```python
from build123d import *

# Parameters (mm, degrees)
F3_D     = 2
F3_DEPTH = 5
F3_TIP   = 0.600860619
F4_W     = 2
F4_H     = 4
F7_D     = 2.5
F7_DEPTH = 6.5
F7_TIP   = 0.7510757738


with BuildPart() as f1:
    # F0 (on Right) → F1 (revolve)
    with BuildSketch(Plane.YZ):
        Polygon((5, 47), (0, 47), (0, 23), (3, 23), (3, 25), (8, 25), (8, 32), (20, 32), (20, 47), (15, 47), (15, 42), (10, 42), align=None)
    revolve(axis=Axis((0, 13.034472242, 0), (0, 1, 0)))

    # F3
    with Locations(Plane(origin=(0, 8, 0), x_dir=(-1, 0, 0), z_dir=(0, 1, 0))):
        with Locations((0, 28.5), (24.6817240079, -14.25), (-24.6817240079, -14.25)):
            Hole(F3_D / 2, depth=F3_DEPTH)
            with Locations((0, 0, -(F3_DEPTH + F3_TIP / 2))):  # 118° drill point
                Cone(0, F3_D / 2, F3_TIP, mode=Mode.SUBTRACT)

    # F4 (on Right) → F5 (revolve)
    with BuildSketch(Plane.YZ):
        with Locations((-1, 45)):
            Rectangle(F4_W, F4_H)
    revolve(axis=Axis((0, -7.9047670588, 0), (0, -1, 0)))

    # F7
    with Locations(Plane.XZ):
        with Locations((0, 37.5), (32.4759526419, -18.75), (-32.4759526419, -18.75)):
            Hole(F7_D / 2, depth=F7_DEPTH)
            with Locations((0, 0, -(F7_DEPTH + F7_TIP / 2))):  # 118° drill point
                Cone(0, F7_D / 2, F7_TIP, mode=Mode.SUBTRACT)


solid = f1.part
```
Source: CAD feature listing. Evaluate the final solid. Frame: model axes, mm. A direction names the side the tool comes from. Coordinates: 2 decimals unless noted, no trailing zeros. Loops run counter-clockwise (first coordinate to the right, second up) from the corner with the lowest first, then second, coordinate; pieces in that order, holes last. Notation, with made-up numbers: (-23.75, -9.5) -> (32.25, -9.5) arc R25 cw to (32.25, 26.5) -> close; hole circle Ø8 at (-34.75, 23.5). An arc over 180 degrees is marked (long way). One line per item, written item: value. Start each with the question number.
Q1. Set-up query: faces 4 (the face through (-14.12, 1.55, 44.83)), 5 (the face through (-31, 20, -10)), 6 (the face through (-33.668, 3.296, -18.375)), 7 (the face through (-31.24, 14.08, -6.94)), 8 (the face through (12.62, 12.46, 40.06)). Return all of +Z, -Z, +X, -X, +Y, -Y with unobstructed straight access to the full face (end or side cutting, diameter ignored); none if empty.
Q2. Section query A-A, the plane z = 0. Return the cut outline in (x, y).
Q3. Mould query, pull axis X, two halves, no side actions, for faces 1 (the face through (-24, 15, -35)), 2 (the face through (12.71, 9.687, 40.359)), 3 (the face through (22.804, 1.521, -2.994)). Classes: pulls with the +X half, pulls with the -X half, needs draft (parallel to the pull), parting line crosses it, or undercut.
Q4. Contact query for flat-ended pins moving along their axis: P1, Ø3, axis at x = 0, z = 37.5, coming from the -Y side; P2, Ø12, axis at x = -36, y = 17.5, coming from the -Z side; P3, Ø1.6, axis at x = 0, z = 28.5, coming from the +Y side; P4, Ø5, axis at x = -15.5, z = -9.5, coming from the +Y side. Output: stop coordinate, or through.
Q5. Line query: line 1 along X through (y, z) = (1.15, 0); line 2 along X through (y, z) = (-0.6, 0); line 3 along X through (y, z) = (5, -18.75). Output: solid intervals per line, ascending.
Results:
1. face 4: +Y, -Y
1. face 5: +Z, -Z, +X, -X, +Y
1. face 6: -Y
1. face 7: +Y
1. face 8: none
2. outline: (-47, -2) -> (-43, -2) -> (-43, 0) -> (-23, 0) -> (-23, 3) -> (-25, 3) -> (-25, 8) -> (-32, 8) -> (-32, 20) -> (-47, 20) -> (-47, 15) -> (-42, 15) -> (-42, 10) -> (-47, 5) -> close; (23, 0) -> (43, 0) -> (43, -2) -> (47, -2) -> (47, 5) -> (42, 10) -> (42, 15) -> (47, 15) -> (47, 20) -> (32, 20) -> (32, 8) -> (25, 8) -> (25, 3) -> (23, 3) -> close
3. face 1: needs draft
3. face 2: parting line crosses it
3. face 3: undercut
4. P1: y = 0
4. P2: z = -36.18
4. P3: y = 2.88
4. P4: through
5. line 1: -47 to -23, 23 to 47
5. line 2: -47 to -43, 43 to 47
5. line 3: -43.1 to -33.73, -31.23 to -16.54, 16.54 to 31.23, 33.73 to 43.1
